The listing builds one solid part. Answer for the finished solid, in the listing's coordinates (mm). A direction names the side the tool comes from. Coordinates: 2 decimals unless noted, no trailing zeros. Order: outer loops, then holes, each group sorted by start corner. A loop starts at its lowest first (then second) coordinate and runs counter-clockwise, first axis right, second up. Notation, with made-up numbers: (-11, -6.75) -> (18, -6.75) arc R11 ccw to (18, 3.25) -> close; hole circle Ø3 at (-18, 77). An arc over 180 degrees is marked (long way). Return JSON: item names as keys, results as strings.
```python
from build123d import *

# Parameters (mm, degrees)
F0_R        = 9.525
F1_DEPTH    = 76.2
F2_DEPTH    = 10.16
F3_T4_DEPTH = 600.435352042
F3_S5_R     = 138.2955463349
F3_T6_DEPTH = 303


# Not quite as in the source:
# - a fillet or chamfer that OpenCascade refuses, or shapes differently, is made with other operations: its cross-section is extruded or revolved along the edge and cut away or added


with BuildPart() as f1:
    # F0 (on Front) → F1 (new body)
    with BuildSketch(Plane.XZ):
        with BuildLine():
            ThreePointArc((28.1677821814, -135.396581135), (107.2873174282, -87.2644810626), (138.2955463349, 0))
            ThreePointArc((138.2955463349, 0), (107.2890589283, 87.2623399316), (28.1731863292, 135.3954567484))
            ThreePointArc((28.1731863292, 135.3954567484), (0, 138.2955463349), (-28.1731863292, 135.3954567484))
            ThreePointArc((-28.1731863292, 135.3954567484), (-138.2955463073, -0.0027599392), (-28.1677821814, -135.396581135))
            ThreePointArc((-28.1677821814, -135.396581135), (0, -138.2955463349), (28.1677821814, -135.396581135))
        make_face()
        with BuildLine():
            ThreePointArc((-35.4519361343, 21.4876397772), (0, 41.4554995009), (35.4519361343, 21.4876397772))
            Line((35.4519361343, 21.4876397772), (85.9505591086, 21.4876397772))
            Line((85.9505591086, 21.4876397772), (85.9505591086, -21.4876397772))
            Line((85.9505591086, -21.4876397772), (35.4519361343, -21.4876397772))
            ThreePointArc((35.4519361343, -21.4876397772), (0, -41.4554995009), (-35.4519361343, -21.4876397772))
            Line((-35.4519361343, -21.4876397772), (-85.9505591086, -21.4876397772))
            Line((-85.9505591086, -21.4876397772), (-85.9505591086, 21.4876397772))
            Line((-85.9505591086, 21.4876397772), (-35.4519361343, 21.4876397772))
        make_face(mode=Mode.SUBTRACT)
        with BuildLine():
            ThreePointArc((28.1731863292, 135.3954567484), (107.2890589283, 87.2623399316), (138.2955463349, 0))
            ThreePointArc((138.2955463349, 0), (107.2873174282, -87.2644810626), (28.1677821814, -135.396581135))
            Line((28.1677821814, -135.396581135), (555.0553956372, -25.7833589585))
            ThreePointArc((555.0553956372, -25.7833589585), (528.9648763124, -0.0553010475), (554.9447987454, 25.7844317855))
            Line((554.9447987454, 25.7844317855), (28.1731863292, 135.3954567484))
        make_face()
        with BuildLine():
            Line((564.856504828, 23.7219966861), (554.9447987454, 25.7844317855))
            ThreePointArc((554.9447987454, 25.7844317855), (528.9648763124, -0.0553010475), (555.0553956372, -25.7833589585))
            Line((555.0553956372, -25.7833589585), (564.7527625578, -23.7659275222))
            ThreePointArc((564.7527625578, -23.7659275222), (576.2301870088, -14.2644938792), (580.5351524758, 0))
            ThreePointArc((580.5351524758, 0), (576.2612979363, 14.2175342345), (564.856504828, 23.7219966861))
        make_face()
        with Locations((554.7499847432, 0)):
            Circle(F0_R, mode=Mode.SUBTRACT)
    extrude(amount=F1_DEPTH)

    # F0 (on Front) → F2 (join)
    with BuildSketch(Plane.XZ):
        with BuildLine():
            ThreePointArc((-28.1677821814, -135.396581135), (-138.2955463073, -0.0027599392), (-28.1731863292, 135.3954567484))
            Line((-28.1731863292, 135.3954567484), (-554.9447987454, 25.7844317855))
            ThreePointArc((-554.9447987454, 25.7844317855), (-536.5861255267, 18.3016145015), (-528.9648170106, 0))
            ThreePointArc((-528.9648170106, 0), (-536.6254184882, -18.3405281566), (-555.0553956372, -25.7833589585))
            Line((-555.0553956372, -25.7833589585), (-28.1677821814, -135.396581135))
        make_face()
        with BuildLine():
            ThreePointArc((-528.9648170106, 0), (-536.5861255267, 18.3016145015), (-554.9447987454, 25.7844317855))
            Line((-554.9447987454, 25.7844317855), (-564.856504828, 23.7219966861))
            ThreePointArc((-564.856504828, 23.7219966861), (-580.5350909463, -0.056330225), (-564.7527625578, -23.7659275222))
            Line((-564.7527625578, -23.7659275222), (-555.0553956372, -25.7833589585))
            ThreePointArc((-555.0553956372, -25.7833589585), (-536.6254184882, -18.3405281566), (-528.9648170106, 0))
        make_face()
        with Locations((-554.7499847432, 0)):
            Circle(F0_R, mode=Mode.SUBTRACT)
    extrude(amount=F2_DEPTH)

    # F3: chamfer of 5.08 on 1 edges, made by hand


with BuildPart() as f3_tool2:
    # F3_s3 → F3_t4 (new body)
    with BuildSketch(Plane(origin=(38.3705740236, 0, 7.9841772943), x_dir=(0, 1, 0), z_dir=(-0.9790297688, 0, -0.2037172351))):
        Polygon((-5.08, -138.2955463349), (-10.16, -133.2155463349), (-10.16, -138.2955463349), align=None)
    extrude(amount=F3_T4_DEPTH)

    # F3_s5 → F3_t6 (cut, symmetric)
    with BuildSketch(Plane.XZ.offset(7.6)):
        Circle(F3_S5_R)
    extrude(amount=F3_T6_DEPTH, both=True, mode=Mode.SUBTRACT)


with BuildPart() as f1_1:
    add(f1.part)

    # F3_t1: cut F3_tool2
    add(f3_tool2.part, mode=Mode.SUBTRACT)


solid = f1_1.part
```
Item 1: Which of the six approach directions +Z, -Z, +X, -X, +Y, -Y give full straight-line access (tool end or side, diameter ignored) to faces 1 (the flat face through (136, -76.2, 2)), 2 (the flat face through (-85.951, -38, 0))?
Answer list:
{"face 1": "+Z, -Z, +X, -X, -Y", "face 2": "+Y, -Y"}
Item 2: The part is cut by section B-B on z = -119.5. Determine the outline of the cut face in (x, y).
Answer list:
{"outline": "(-104.58, -10.16) -> (-69.61, -10.16) -> (-69.61, -76.2) -> (104.58, -76.2) -> (104.58, 0) -> (-104.58, 0) -> close"}
Item 3: The part is cut by section D-D on z = 69. Determine the outline of the cut face in (x, y).
Answer list:
{"outline": "(-347.26, -5.08) -> (-322.32, -10.16) -> (-119.85, -10.16) -> (-119.85, -76.2) -> (347.26, -76.2) -> (347.26, 0) -> (-347.26, 0) -> close"}
Item 4: The part is cut by section C-C on x = 408.5. Determine the outline of the cut face in (y, z), plus the area to 3 significant figures.
Answer list:
{"outline": "(-76.2, -56.27) -> (0, -56.27) -> (0, 56.26) -> (-76.2, 56.26) -> close", "area": "8,570 mm2"}
Item 5: Determine the mould class of faces 3 (the flat face through (-297.54, -7.58, 76.79)), 4 (the flat face through (-8, 0, -60)), 5 (the flat face through (-61, -38, 21.488)) for opening direction Z: pulls with the +Z half, pulls with the -Z half, needs draft (parallel to the pull), parting line crosses it, or undercut.
Answer list:
{"face 3": "pulls with the +Z half", "face 4": "needs draft", "face 5": "undercut"}
Item 6: The part is cut by section A-A on y = -41. Count the separate pieces of the cut face and the enclosed holes in it, plus the area to 3 significant figures.
Answer list:
{"separate pieces": "1", "enclosed holes": "2", "area": "114,000 mm2"}
Item 7: Flat-ended cylindrical pins translate along their axes: pin 1 (1 mm diameter, centred on y = -49, z = 78, fed in from -X); pin 2 (5 mm diameter, centred on x = -10, y = -8, fed in from -Z); pin 3 (2 mm diameter, centred on y = -44.5, z = 24, fed in from -X). Find the tip coordinate at first contact, or state that the pin passes through.
Answer list:
{"pin 1": "x = -114.54", "pin 2": "z = -138.09", "pin 3": "x = -136.37"}
Item 8: Find the intervals of material crossed by probe 1 along X at (y, z) = (-72, -2); probe 2 along Z at (x, y) = (55.5, -46.5); probe 3 along Y at (x, z) = (-311, 19), in increasing order.
Answer list:
{"probe 1": "-138.28 to -85.95, 85.95 to 545.44, 564.06 to 580.46", "probe 2": "-129.71 to -21.49, 21.49 to 129.71", "probe 3": "-10.16 to 0"}
